Read the model definition and answer for the solid it produces. Units are mm, in the model's axes. A direction names the side the tool comes from. Coordinates: 2 decimals unless noted, no trailing zeros. Order: outer loops, then holes, each group sorted by start corner. A loop starts at its lowest first (then second) coordinate and runs counter-clockwise, first axis right, second up. Notation, with made-up numbers: M 73.5,9 L 100.5,9 A16 ccw 100.5,28 Z; hole C 4.5,-38.5 d8. An arc over 180 degrees is marked long. Write each question's results on one line, items separated by ' | '.
```python
from build123d import *

# Parameters (mm, degrees)
ESQUISSE1_W               = 75
ESQUISSE1_H               = 60
BOSS_EXTRU_1_DEPTH        = 8
ESQUISSE2_W               = 40
ESQUISSE2_H               = 20
ENL_V_MAT_EXTRU_1_DEPTH   = 8
ESQUISSE3_W               = 8.5
ESQUISSE3_H               = 2.5
ENL_V_MAT_EXTRU_2_DEPTH   = 8
ESQUISSE4_R               = 2.7
ENL_V_MAT_EXTRU_3_DEPTH   = 49.685213361
SYM_TRIE4_COPY_1_SKETCH_W = 8.5
SYM_TRIE4_COPY_1_SKETCH_H = 2.5
SYM_TRIE4_COPY_1_DEPTH    = 8
SYM_TRIE4_COPY_2_SKETCH_R = 2.7
SYM_TRIE4_COPY_2_DEPTH    = 49.685213361
ESQUISSE6_W               = 75
ESQUISSE6_H               = 60
BOSS_EXTRU_2_DEPTH        = 35
ESQUISSE7_W               = 65
ESQUISSE7_H               = 50
ENL_V_MAT_EXTRU_4_DEPTH   = 35


with BuildPart() as part:
    # Esquisse1 → Boss.-Extru.1 (new body)
    with BuildSketch(Plane.XY):
        Rectangle(ESQUISSE1_W, ESQUISSE1_H)
    extrude(amount=-BOSS_EXTRU_1_DEPTH)

    # Esquisse2 → Enlèv. mat.-Extru.1 (cut)
    with BuildSketch(Plane.XY):
        with Locations((0, 12.5)):
            Rectangle(ESQUISSE2_W, ESQUISSE2_H)
    enl_v_mat_extru_1 = extrude(amount=-ENL_V_MAT_EXTRU_1_DEPTH, mode=Mode.SUBTRACT)

    # Esquisse3 → Enlèv. mat.-Extru.2 (cut)
    with BuildSketch(Plane.XY):
        with Locations((-24.25, 12.5)):
            Rectangle(ESQUISSE3_W, ESQUISSE3_H)
    enl_v_mat_extru_2 = extrude(amount=-ENL_V_MAT_EXTRU_2_DEPTH, mode=Mode.SUBTRACT)

    # Esquisse4 → Enlèv. mat.-Extru.3 (cut, through all)
    with BuildSketch(Plane.XY):
        with Locations((-24, 17.5)):
            Circle(ESQUISSE4_R)
        with Locations((-24, 7.5)):
            Circle(ESQUISSE4_R)
    enl_v_mat_extru_3 = extrude(amount=-ENL_V_MAT_EXTRU_3_DEPTH, mode=Mode.SUBTRACT)

    # Symétrie2: Enlèv. mat.-Extru.2, Enlèv. mat.-Extru.3 across plane
    add(enl_v_mat_extru_2.mirror(Plane(origin=(0, 0, 0), x_dir=(0, 0, 1), z_dir=(1, 0, 0))), mode=Mode.SUBTRACT)
    add(enl_v_mat_extru_3.mirror(Plane(origin=(0, 0, 0), x_dir=(0, 0, 1), z_dir=(1, 0, 0))), mode=Mode.SUBTRACT)

    # Symétrie4: Enlèv. mat.-Extru.1, Enlèv. mat.-Extru.2, Enlèv. mat.-Extru.3 across plane
    add(enl_v_mat_extru_1.mirror(Plane.ZX), mode=Mode.SUBTRACT)
    add(enl_v_mat_extru_2.mirror(Plane.ZX), mode=Mode.SUBTRACT)
    add(enl_v_mat_extru_3.mirror(Plane.ZX), mode=Mode.SUBTRACT)

    # Symétrie4 copy 1 sketch → Symétrie4 copy 1 (cut)
    with BuildSketch(Plane(origin=(0, 0, 0), x_dir=(-1, 0, 0), z_dir=(0, 0, 1))):
        with Locations((-24.25, 12.5)):
            Rectangle(SYM_TRIE4_COPY_1_SKETCH_W, SYM_TRIE4_COPY_1_SKETCH_H)
    extrude(amount=-SYM_TRIE4_COPY_1_DEPTH, mode=Mode.SUBTRACT)

    # Symétrie4 copy 2 sketch → Symétrie4 copy 2 (cut, through all)
    with BuildSketch(Plane(origin=(0, 0, 0), x_dir=(-1, 0, 0), z_dir=(0, 0, 1))):
        with Locations((-24, 17.5)):
            Circle(SYM_TRIE4_COPY_2_SKETCH_R)
        with Locations((-24, 7.5)):
            Circle(SYM_TRIE4_COPY_2_SKETCH_R)
    extrude(amount=-SYM_TRIE4_COPY_2_DEPTH, mode=Mode.SUBTRACT)

    # Esquisse6 → Boss.-Extru.2 (add)
    with BuildSketch(Plane.XY):
        Rectangle(ESQUISSE6_W, ESQUISSE6_H)
    extrude(amount=BOSS_EXTRU_2_DEPTH)

    # Esquisse7 → Enlèv. mat.-Extru.4 (cut)
    with BuildSketch(Plane.XY.offset(35)):
        Rectangle(ESQUISSE7_W, ESQUISSE7_H)
    extrude(amount=-ENL_V_MAT_EXTRU_4_DEPTH, mode=Mode.SUBTRACT)


solid = part.part
```
(1) Straight lines are drawn through the part: line 1 (Y direction, x = 10.5, z = -5); line 2 (X direction, y = -7.5, z = -3.25); line 3 (X direction, y = -1, z = 1). For each, find the intervals that lie inside material, in ascending order.
Conclusion:
line 1: -30 to -22.5, -2.5 to 2.5, 22.5 to 30 | line 2: -37.5 to -26.7, -21.3 to -20, 20 to 21.3, 26.7 to 37.5 | line 3: -37.5 to -32.5, 32.5 to 37.5
(2) The part is cut by section B-B, the plane y = 7.5. Write down the section's boundary in (x, z), then the cut area to 3 significant figures.
Conclusion:
outline: M -37.5,-8 L -26.7,-8 L -26.7,0 L -32.5,0 L -32.5,35 L -37.5,35 Z; M -21.3,-8 L -20,-8 L -20,0 L -21.3,0 Z; M 20,-8 L 21.3,-8 L 21.3,0 L 20,0 Z; M 26.7,-8 L 37.5,-8 L 37.5,35 L 32.5,35 L 32.5,0 L 26.7,0 Z | area: 544 mm²
(3) The part is cut by section D-D, the plane z = 1. Write down the section's boundary in (x, y).
Conclusion:
outline: M -37.5,-30 L 37.5,-30 L 37.5,30 L -37.5,30 Z; hole M -32.5,-25 L 32.5,-25 L 32.5,25 L -32.5,25 Z
(4) The mould has two halves that part along X. Classify faces 1 (the cylindrical face through (-24.351, 20.177, -3.944)), 2 (the flat face through (-1, 30, 13)), 3 (the flat face through (37.5, 0, 13)): pulls with the +X half, pulls with the -X half, needs draft (parallel to the pull), parting line crosses it, or undercut.
Conclusion:
face 1: undercut | face 2: needs draft | face 3: pulls with the +X half
(5) For faces 4 (the flat face through (-1, -30, 13)), 5 (the flat face through (0, -25, 18)), 6 (the flat face through (0, -22.5, -4)), determine the directions among +Z, -Z, +X, -X, +Y, -Y from which every point of the face is accessible in a straight line to the end or side of a thin tool.
Conclusion:
face 4: +Z, -Z, +X, -X, -Y | face 5: +Z | face 6: +Z, -Z
(6) The part is cut by section A-A, the plane x = 5. Write down the section's boundary in (y, z).
Conclusion:
outline: M -30,-8 L -22.5,-8 L -22.5,0 L -25,0 L -25,35 L -30,35 Z; M -2.5,-8 L 2.5,-8 L 2.5,0 L -2.5,0 Z; M 22.5,-8 L 30,-8 L 30,35 L 25,35 L 25,0 L 22.5,0 Z
(7) Given pin 1 (6 mm diameter, centred on x = 24, y = -17.5, fed in from +Z), flat-ended and moving along its own axis, determine where the tip first touches the part or whether it passes through.
Conclusion:
pin 1: z = 0
(8) The part is cut by section C-C, the plane x = -24. Count the separate pieces of the cut face and the enclosed holes in it, then the cut area to 3 significant figures.
Conclusion:
separate pieces: 7 | enclosed holes: 0 | area: 617 mm²
